Work out the finished part from the listing and answer in its coordinate system (mm). A direction names the side the tool comes from. Give positions to 0.01 mm unless a question says otherwise; leave off trailing zeros. Order: outer loops, then holes, each group sorted by start corner. A loop starts at its lowest first (then second) coordinate and runs counter-clockwise, first axis right, second up. Notation, with made-up numbers: (22.5, 87.5) -> (56.5, 87.5) arc R24 cw to (56.5, 114.5) -> close; hole circle Ø11 at (-2, 89.5). An arc over 180 degrees is marked (long way). Use a Markdown table: item, result. Add a question column.
```python
from build123d import *

# Parameters (mm, degrees)
BOSS_EXTRUDE1_DEPTH = 2.5
SKETCH2_R           = 1.5
CUT_EXTRUDE1_DEPTH  = 10
SKETCH3_W           = 124.34
SKETCH3_H           = 2.5
CUT_EXTRUDE2_DEPTH  = 1
SKETCH4_W           = 2.5
SKETCH4_H           = 33.25
BOSS_EXTRUDE2_DEPTH = 2
FILLET2_R           = 10


with BuildPart() as part:
    # Sketch1 → Boss-Extrude1 (new body)
    with BuildSketch(Plane.XY):
        Polygon((-67.40224359, 38.860576923), (-67.40224359, 4.610576923), (56.93775641, 4.610576923), (56.93775641, -17.519423077), (67.94775641, -17.519423077), (67.94775641, 38.860576923), align=None)
    extrude(amount=BOSS_EXTRUDE1_DEPTH)

    # Sketch2 → Cut-Extrude1 (cut)
    with BuildSketch(Plane(origin=(0, 0, 0), x_dir=(-1, 0, 0), z_dir=(0, 0, -1))):
        with Locations((-27.399068165, 14.110576923)):
            Circle(SKETCH2_R)
        with Locations((38.600931835, 14.110576923)):
            Circle(SKETCH2_R)
    extrude(amount=-CUT_EXTRUDE1_DEPTH, mode=Mode.SUBTRACT)

    # Sketch3 → Cut-Extrude2 (cut)
    with BuildSketch(Plane.XZ.offset(-4.610576923)):
        with Locations((-5.23224359, 1.25)):
            Rectangle(SKETCH3_W, SKETCH3_H)
    extrude(amount=-CUT_EXTRUDE2_DEPTH, mode=Mode.SUBTRACT)

    # Sketch4 → Boss-Extrude2 (add)
    with BuildSketch(Plane.ZY.offset(67.40224359)):
        with Locations((1.25, 22.235576923)):
            Rectangle(SKETCH4_W, SKETCH4_H)
    extrude(amount=BOSS_EXTRUDE2_DEPTH)

    # Fillet2
    fillet2_edges = [part.edges().sort_by_distance(p)[0] for p in [
        (-69.40224359, 38.860576923, 1.25),
    ]]
    fillet(fillet2_edges, radius=FILLET2_R)


solid = part.part
```
1) Straight lines are drawn through the part: line 1 (Y direction, x = 21, z = 1.9); line 2 (X direction, y = 15, z = 2.25); line 3 (X direction, y = 3.5, z = 0.75). For each, find the intervals that lie inside material, in ascending order.
2) The part is cut by section B-B, the plane x = 35.5. Determine the outline of the cut face in (y, z).
3) The part is cut by section A-A, the plane z = 1.3. Determine the outline of the cut face in (x, y), then the cut area to 3 significant figures.
4) Determine the mould class of faces 3 (the cylindrical face through (25.97, 14.56, 1.23)), 4 (the flat face through (0, 23, 0)), 5 (the flat face through (67.948, 10, 1)) for opening direction X: released by +X, released by -X, zero draft, split by the parting line, or undercut.
5) Which of the six approach directions +Z, -Z, +X, -X, +Y, -Y give full straight-line access (tool end or side, diameter ignored) to faces 1 (the cylindrical face through (-40.03, 14.56, 1.23)), 2 (the flat face through (-5, 5.611, 1))?
6) The part is cut by section C-C, the plane y = 1. Determine the outline of the cut face in (x, z), then the cut area to 3 significant figures.
7) Flat-ended cylindrical pins translate along their axes: pin 1 (1.8 mm diameter, centred on x = 27.4, y = 14.11, fed in from -Z); pin 2 (1.2 mm diameter, centred on y = -3.5, z = 0.5, fed in from -X). Find the tip coordinate at first contact, or state that the pin passes through.
A:
| question | item | result |
|---|---|---|
| 1 | line 1 | 5.61 to 38.86 |
| 1 | line 2 | -69.4 to -39.81, -37.39 to 26.19, 28.61 to 67.95 |
| 1 | line 3 | 56.94 to 67.95 |
| 2 | outline | (5.61, 0) -> (38.86, 0) -> (38.86, 2.5) -> (5.61, 2.5) -> close |
| 3 | outline | (-69.4, 5.61) -> (56.94, 5.61) -> (56.94, -17.52) -> (67.95, -17.52) -> (67.95, 38.86) -> (-59.4, 38.86) arc R10 ccw to (-69.4, 28.86) -> close; hole circle Ø3 at (-38.6, 14.11); hole circle Ø3 at (27.4, 14.11) |
| 3 | area | 4,790 mm^2 |
| 4 | face 3 | undercut |
| 4 | face 4 | zero draft |
| 4 | face 5 | released by +X |
| 5 | face 1 | +Z, -Z |
| 5 | face 2 | +Z, -Z, -X, -Y |
| 6 | outline | (56.94, 0) -> (67.95, 0) -> (67.95, 2.5) -> (56.94, 2.5) -> close |
| 6 | area | 27.5 mm^2 |
| 7 | pin 1 | through |
| 7 | pin 2 | x = 56.94 |
